Solid Edge part; units mm, degrees
sketch "Sketch1" plane through (0, 0, 0) normal (0, -1, 0) x (1, 0, 0)
  circle A0 centre (-15.5, 0) radius 1.4
  line L0 (-19, -2.75) -> (-19, 2.75)
  line L1 (-19, 2.75) -> (19, 2.75)
  line L2 (19, 2.75) -> (19, -2.75)
  line L3 (19, -2.75) -> (-19, -2.75)
  circle A1 centre (15.5, 0) radius 1.4
extrude "Protrusion1" add sketch "Sketch1" along normal blind 3
sketch "Sketch2" plane through (0, -3, 0) normal (0, -1, 0) x (1, 0, 0)
  line L0 (12.5, -1.25) -> (-12.5, -1.25)
  line L1 (-12.5, -1.25) -> (-12.5, 1.25)
  line L2 (-12.5, 1.25) -> (12.5, 1.25)
  line L3 (12.5, 1.25) -> (12.5, -1.25)
extrude "ExtrudedProtrusion_2" add sketch "Sketch2" along normal blind 15
sketch "Sketch3" plane through (0, -10.5, 1.25) normal (0, 0, 1) x (1, 0, 0)
  line L0 (-12.5, 7.5) -> (-3.0729, -3.8125)
  arc A0 (-3.0729, -3.8125) -> (3.0729, -3.8125) centre (0, -1.2518) ccw
  line L1 (3.0729, -3.8125) -> (12.5, 7.5)
  line L2 (12.5, -7.5) -> (12.5, 7.5)
  line L3 (-12.5, -7.5) -> (12.5, -7.5)
  line L4 (-12.5, -7.5) -> (-12.5, 7.5)
extrude "ExtrudedCutout_1" cut sketch "Sketch3" against normal blind 25.6069
sketch "Sketch4" plane through (0, -10.5, 1.25) normal (0, 0, 1) x (1, 0, 0)
  circle A0 centre (0, -0.5) radius 2.4
extrude "ExtrudedCutout_2" cut sketch "Sketch4" against normal blind 14.916
fillet "Round_1" radius 3 4 edges at (0, -3, 1.25) (0, -3, -1.25) (12.5, -3, 0) (-12.5, -3, 0)
fillet "Round_2" radius 2 4 edges at (-19, -1.5, 2.75) (-19, -1.5, -2.75) (19, -1.5, -2.75) (19, -1.5, 2.75)
properties material "PLA"
Geometry: final body of the model. Coordinates: model frame, mm. A direction names the side the tool comes from. Round coordinates to 2 decimals unless told otherwise and drop trailing zeros. Order: outer loops, then holes, each group sorted by start corner. A loop starts at its lowest first (then second) coordinate and runs counter-clockwise, first axis right, second up. Notation, with made-up numbers: (-21.5, 51) -> (35.5, 51) arc R32 ccw to (35.5, 90) -> close; hole circle Ø9 at (85.25, 74.5). An arc over 180 degrees is marked (long way). Use one line per item in the form item = value. Start each with the question number.
1. Line query: probe 1 along Y at (x, z) = (0, -0.1); probe 2 along Z at (x, y) = (15.5, -2.25); probe 3 along X at (y, z) = (-11.25, -0.85) (3 decimals). Output: solid intervals per line, ascending.
2. Draft query along X for faces 4 (the face through (12.6, -3.3, 0)), 5 (the face through (0, -8, 1.25)), 6 (the face through (1.29, -8.976, 0.018)), 7 (the face through (-16.9, -1.48, -0.06)). Return one class per face: pulls with the +X half, pulls with the -X half, needs draft (parallel to the pull), parting line crosses it, or undercut.
3. Cut plane D-D (y = -10.25). Return the cut outline in (x, z).
4. Pin query (flat end, axial travel): pin 1 Ø1 at (x, z) = (-6, 2) entering from -Y; pin 2 Ø2 at (x, z) = (-6, -1.5) entering from -Y; pin 3 Ø2 at (x, z) = (3.5, 0) entering from -Y; pin 4 Ø6 at (x, y) = (0.5, -4) entering from -Z. Return the tip coordinate at first contact, or that it passes through.
5. Reachability of faces 1 (the face through (0, -8, -1.25)), 2 (the face through (-17, -3, 1)), 3 (the face through (7.4, -9.12, 0.02)) from +Z, -Z, +X, -X, +Y, -Y: full face, straight path, thin tool, end or side. Return the list, or none.
6. Cut plane C-C (x = 0). Return the cut outline in (y, z), then the cut area to 3 significant figures.
7. Cut plane B-B (z = 0). Return the cut outline in (x, y), then the cut area to 3 significant figures.
8. Cut plane A-A (x = 15.5). Return the cut outline in (y, z), then the cut area to 3 significant figures.
Solution:
q1.probe_1 = -15.75 to -13.4, -8.6 to 0
q1.probe_2 = -2.75 to -1.4, 1.4 to 2.75
q1.probe_3 = -5.625 to -2.387, 2.387 to 5.625
q2.face_4 = pulls with the +X half
q2.face_5 = needs draft
q2.face_6 = undercut
q2.face_7 = undercut
q3.outline = (-6.46, -1.25) -> (-2.28, -1.25) -> (-2.28, 1.25) -> (-6.46, 1.25) -> close; (2.28, -1.25) -> (6.46, -1.25) -> (6.46, 1.25) -> (2.28, 1.25) -> close
q4.pin_1 = -4.4
q4.pin_2 = -11.96
q4.pin_3 = -14.87
q4.pin_4 = -2.75
q5.face_1 = -Z, +X, -X, -Y
q5.face_2 = +Z, -Z, -X, -Y
q5.face_3 = +Z, -Z, +X, -Y
q6.outline = (-15.75, -1.25) -> (-13.4, -1.25) -> (-13.4, 1.25) -> (-15.75, 1.25) -> close; (-8.6, -1.25) -> (-5.6, -1.25) arc R3 cw to (-3, -2.75) -> (0, -2.75) -> (0, 2.75) -> (-3, 2.75) arc R3 cw to (-5.6, 1.25) -> (-8.6, 1.25) -> close
q6.area = 38.6 mm^2
q7.outline = (-19, -3) -> (-16.9, -3) -> (-16.9, 0) -> (-19, 0) -> close; (-14.1, -3) -> (-13.91, -3) arc R3 cw to (-11.6, -4.08) -> (-3.07, -14.31) arc R4 ccw to (3.07, -14.31) -> (11.6, -4.08) arc R3 cw to (13.91, -3) -> (14.1, -3) -> (14.1, 0) -> (-14.1, 0) -> close; (16.9, -3) -> (19, -3) -> (19, 0) -> (16.9, 0) -> close; hole circle Ø4.8 at (0, -11)
q7.area = 262 mm^2
q8.outline = (-3, -2.75) -> (0, -2.75) -> (0, -1.4) -> (-3, -1.4) -> close; (-3, 1.4) -> (0, 1.4) -> (0, 2.75) -> (-3, 2.75) -> close
q8.area = 8.10 mm^2
